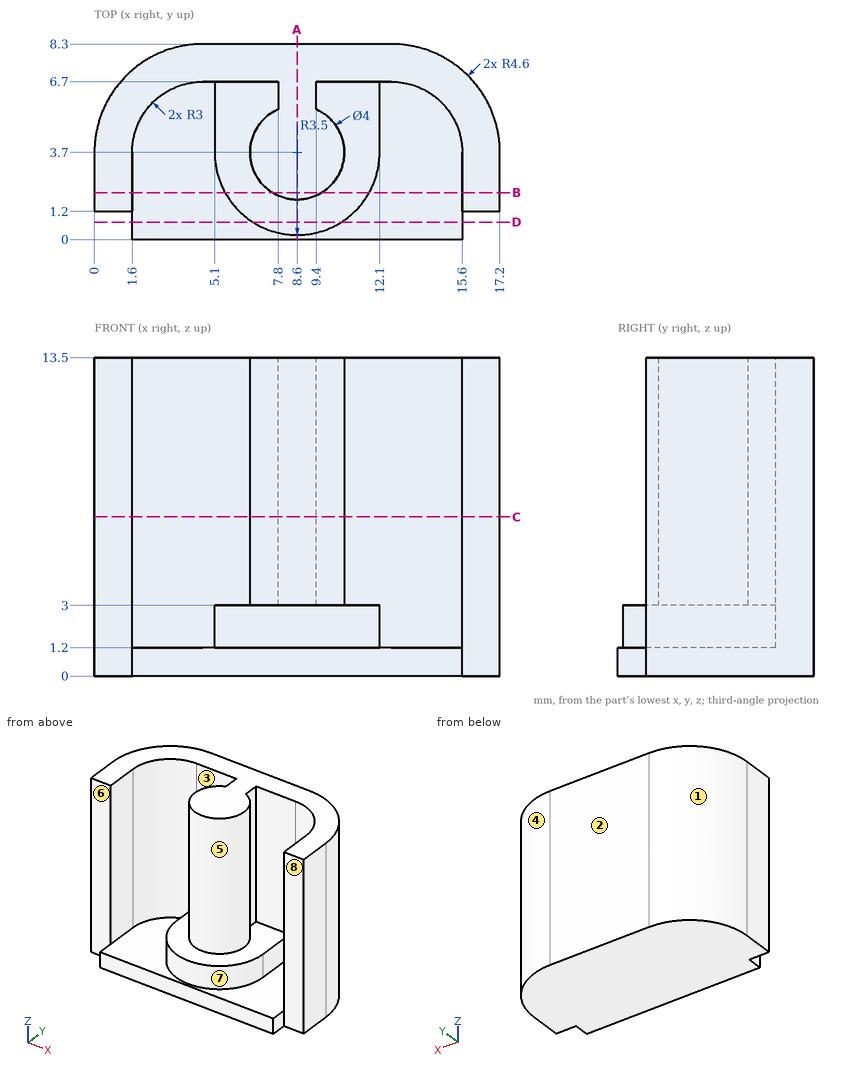
Design review of the part shown in the three views and the two pictorial views. Dimensions are in mm from the part's minimum x, y and z. A direction names the side the tool comes from. Round coordinates to 2 decimals unless told otherwise and drop trailing zeros. Write each loop counter-clockwise with the first axis right and the second up, starting at its lowest first coordinate (ties: lowest second). Pieces come first, ordered by that corner, then holes. Notation, with made-up numbers: (75, -23) - (86, -23) arc R11 ccw to (86, -5) - close; hole circle Ø1 at (81, 89). An arc over 180 degrees is marked (long way). Answer as CSV lines item,"result". Start each with the question number.
(1) Add section D-D, the plane y = 0.75. State the section outline as (x, z) points.
(2) Add section B-B, the plane y = 2. State the section outline as (x, z) points.
(3) For pin 1 (1 mm diameter, centred on x = 6, z = 6, fed in from -Y); pin 2 (1.3 mm diameter, centred on y = 0.5, z = 1, fed in from -X); pin 3 (1.3 mm diameter, centred on y = 6, z = 7, fed in from +X), all flat-tipped, find the tip position at first contact; note any pin that passes through.
(4) For line 1 (X direction, y = 5.75, z = 6); line 2 (X direction, y = 3.5, z = 5); line 3 (Z direction, x = 5.5, y = 4.5), list the stretches that pass through material, from the lowest coordinate up.
(5) Machinability: for the marked faces 5, 6, 7 and 8, which of the approach directions +Z, -Z, +X, -X, +Y, -Y give a long, thin tool a straight path to every point of the face, cutting with its end or side? Answer none if there is none.
(6) Mouldability with a two-part tool opening along X and no side actions: class the marked faces 1, 2, 3 and 4 as +X half, -X half, draft (parallel to the pull), parting line (faces both ways), or undercut.
(7) Add section C-C, the plane z = 6.75. State the section outline as (x, y) points, plus the area to 3 significant figures.
(8) Add section A-A, the plane x = 8.6. State the section outline as (y, z) points, plus the area to 3 significant figures.
From the geometry:
1,outline,"(1.6, 0) - (15.6, 0) - (15.6, 1.2) - (10.48, 1.2) - (10.48, 3) - (6.72, 3) - (6.72, 1.2) - (1.6, 1.2) - close"
2,outline,"(0, 0) - (17.2, 0) - (17.2, 13.5) - (15.6, 13.5) - (15.6, 1.2) - (11.66, 1.2) - (11.66, 3) - (9.65, 3) - (9.65, 13.5) - (7.55, 13.5) - (7.55, 3) - (5.54, 3) - (5.54, 1.2) - (1.6, 1.2) - (1.6, 13.5) - (0, 13.5) - close"
3,pin 1,"stops at y = 6.7"
3,pin 2,"stops at x = 1.6"
3,pin 3,"stops at x = 16.89"
4,line 1,"x = 0.48 to 2.41, 7.8 to 9.4, 14.79 to 16.72"
4,line 2,"x = 0 to 1.6, 6.61 to 10.59, 15.6 to 17.2"
4,line 3,"z = 0 to 3"
5,face 5,"+Z"
5,face 6,"+Z, -Z, -X, -Y"
5,face 7,"+Z, -Y"
5,face 8,"+Z, -Z, +X, -Y"
6,face 1,"-X half"
6,face 2,"draft"
6,face 3,"undercut"
6,face 4,"+X half"
7,outline,"(0, 1.2) - (1.6, 1.2) - (1.6, 3.7) arc R3 cw to (4.6, 6.7) - (7.8, 6.7) - (7.8, 5.53) arc R2 ccw (long way) to (9.4, 5.53) - (9.4, 6.7) - (12.6, 6.7) arc R3 cw to (15.6, 3.7) - (15.6, 1.2) - (17.2, 1.2) - (17.2, 3.7) arc R4.6 ccw to (12.6, 8.3) - (4.6, 8.3) arc R4.6 ccw to (0, 3.7) - close"
7,area,"54.2 mm²"
8,outline,"(0, 0) - (8.3, 0) - (8.3, 13.5) - (1.7, 13.5) - (1.7, 3) - (0.2, 3) - (0.2, 1.2) - (0, 1.2) - close"
8,area,"93.8 mm²"
